For this review, take the finished solid that the model builds, in its own axes (mm). Face numbers are marked on the shaded views. Give positions to 0.01 mm unless a question says otherwise; leave off trailing zeros. Order: outer loops, then holes, each group sorted by start corner. A loop starts at its lowest first (then second) coordinate and runs counter-clockwise, first axis right, second up. Notation, with made-up numbers: (89, -16.75) - (100, -16.75) arc R27 ccw to (100, 17.25) - close; hole circle Ø1 at (47.25, -7.75). An arc over 180 degrees is marked (long way). Use a Markdown table: item, result. Add a question column.
1) Clearance check with flat-ended pins moving along their axes: P1, Ø5, axis at y = 17.5, z = 117.5, coming from the +X side; P2, Ø1, axis at y = 23, z = 14.5, coming from the +X side; P3, Ø4, axis at y = 13.5, z = 117.5, coming from the -X side. State where each tip first meets the part, or that it passes through.
2) We need section C-C on x = 18. Write out the cut boundary in (y, z).
3) We need section D-D on y = 2.5. Write out the cut boundary in (x, z), then the cut area to 3 significant figures.
4) We need section B-B on z = 95. Write out the cut boundary in (x, y), then the cut area to 3 significant figures.
5) Mouldability with a two-part tool opening along Y and no side actions: class the marked faces 1, 2, 3 and 4 as released by +Y, released by -Y, zero draft, split by the parting line, or undercut.
6) We need section A-A on x = 31. Write out the cut boundary in (y, z), then the cut area to 3 significant figures.
7) Wall thickness on L1, parallel to X at y = -12.5, z = 3; L2, parallel to Y at x = 34, z = 69.5; L3, parallel to Y at x = 8, z = 102: over which ranges is each line inside the solid? List them lowest first.
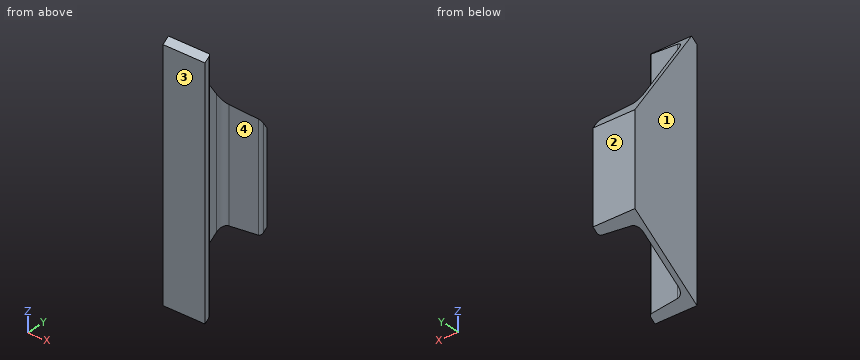
Autodesk Inventor part; units mm, degrees
ref_plane "Начальная плоскость" through (0, 0, -22.1942) normal (0, 0, 1) x (1, 0, 0)
ref_plane "Конечная плоскость" through (0, 0, 186.7165) normal (0, 0, 1) x (1, 0, 0)
ref_plane "РабПлоскость8" through (-29, 0, 205.1172) normal (0, -0.5661745, 0.8242854) x (1, 0, 0)
ref_plane "Начальная плоскость" through (0, 0, -22.1942) normal (0, 0, 1) x (1, 0, 0)
ref_plane "Конечная плоскость" through (0, 0, 186.7165) normal (0, 0, 1) x (1, 0, 0)
sketch "Эскиз" plane through (0, 0, 0) normal (0, 0, 1) x (1, 0, 0)
  line L0 (36, -32.5) -> (0, -32.5)
  line L1 (36, -32.5) -> (36, -28.696)
  line L2 (33.6994, -26.2039) -> (9.9215, -24.3017)
  line L3 (4.4, -18.3208) -> (4.4, 18.3208)
  line L4 (33.6994, 26.2039) -> (9.9215, 24.3017)
  line L5 (36, 28.696) -> (36, 32.5)
  line L6 (0, 32.5) -> (36, 32.5)
  line L7 (0, -32.5) -> (0, 32.5)
  arc A0 (4.4, -18.3208) -> (9.9215, -24.3017) centre (10.4, -18.3208) ccw
  arc A1 (9.9215, 24.3017) -> (4.4, 18.3208) centre (10.4, 18.3208) ccw
  arc A2 (36, -28.696) -> (33.6994, -26.2039) centre (33.5, -28.696) ccw
  arc A3 (33.6994, 26.2039) -> (36, 28.696) centre (33.5, 28.696) ccw
  line L8 (0, 45.5) -> (0, -45.5) construction
  line L9 (-7.2974, 0) -> (43.7847, 0) construction
  point P0 (36, -26.388)
  point P1 (4.4, -23.86)
  point P2 (4.4, 23.86)
  point P3 (36, 26.388)
  dimension "d3" = 36
  dimension "d5" = 4.4
  dimension "d7" = 65
  dimension "d9" = 8.64
  dimension "d11" = 8.64
  dimension "d13" = 6.112
  dimension "d15" = 6.112
  dimension "d22" = 6
  dimension "d23" = 2.5
  dimension "d24" = 32.5
  dimension "d25" = 0
extrude "Тело" add sketch "Эскиз" along normal up to surface (208.9107 mm away) from surface at -22.1942
sketch "Sketch3" plane through (0, 0, 0) normal (0, 0, 1) x (1, 0, 0)
  line L0 (0, 0) -> (10, 0)
ref_plane "Work Plane7" through (0, 0, 0) normal (0, -1, 0) x (1, 0, 0)
sketch "Sketch4" plane through (0, 0, 0) normal (0, -1, 0) x (1, 0, 0)
  line L0 (-2, -22.1942) -> (12, -22.1942)
  line L1 (-2, 186.7165) -> (12, 186.7165)
  dimension "d29" = 208.9107
ref_plane "РабПлоскость8" through (-29, 0, 205.1172) normal (0, -0.5661745, 0.8242854) x (1, 0, 0)
split "Разделение1" plane through (-29, 0, 205.1172) removes the side toward (0, -0.5661745, 0.8242854)
ref_plane "РабПлоскость9" through (36, 328.8626, 224.5798) normal (0, 0.5639457, -0.8258119) x (1, 0, 0)
split "Разделение2" plane through (36, 328.8626, 224.5798) removes the side toward (0, 0.5639457, -0.8258119)
ref_plane "РабПлоскость10" through (36, 68.6864, 46.906) normal (0, 0.8258135, 0.5639433) x (1, 0, 0)
split "Разделение3" plane through (36, 68.6864, 46.906) removes the side toward (0, 0.8258135, 0.5639433)
equation "\"d3\" = b"
equation "\"d7\" = ParH"
equation "\"d22\" = R"
equation "\"d23\" = R1"
equation "\"d24\" = 0.5 * d7"
equation "\"d16\" = G_L"
equation "\"R1\" = 2.5"
equation "\"R\" = 6"
equation "\"t1\" = 4.4"
equation "\"t2\" = 7.2"
equation "\"ParH\" = 65"
equation "\"b\" = 36"
equation "\"msp_x1\" = 0.04 * b"
equation "\"msp_x2\" = -0.08 * t1 + 0.04 * b"
equation "\"G_L\" = d29"
equation "\"ex\" = 0"
equation "\"G_OFFSET_START\" = 22.1942"
equation "\"G_OFFSET_END\" = -18.40074"
equation "\"d26\" = -G_OFFSET_START"
equation "\"d27\" = G_OFFSET_END + B_L"
equation "\"B_L\" = 205.11724"
properties part number "Швеллер 6.5U-208,91 ГОСТ 8240-97" material "Сталь, мягкая"
Checked values:
| question | item | result |
|---|---|---|
| 1 | P1 | x = 4.64 |
| 1 | P2 | through |
| 1 | P3 | x = 0 |
| 2 | outline | (-32.5, -22.19) - (-24.95, -17.04) - (-24.95, 184.02) - (-26.79, 186.72) - (-32.5, 182.79) - close; (24.95, 17.04) - (32.5, 22.19) - (32.5, 99.9) - (24.95, 110.95) - close |
| 3 | outline | (0, 1.71) - (4.4, 1.71) - (4.4, 143.83) - (0, 143.83) - close |
| 3 | area | 625 mm² |
| 4 | outline | (0, -32.5) - (36, -32.5) - (36, -28.7) arc R2.5 ccw to (33.7, -26.2) - (9.92, -24.3) arc R6 cw to (4.4, -18.32) - (4.4, 18.32) arc R6 cw to (9.92, 24.3) - (33.7, 26.2) arc R2.5 ccw to (36, 28.7) - (36, 32.5) - (0, 32.5) - close |
| 4 | area | 763 mm² |
| 5 | face 1 | zero draft |
| 5 | face 2 | released by +Y |
| 5 | face 3 | released by -Y |
| 5 | face 4 | undercut |
| 6 | outline | (-32.5, -22.19) - (-25.99, -17.75) - (-25.99, 185.54) - (-26.79, 186.72) - (-32.5, 182.79) - close; (25.99, 17.75) - (32.5, 22.19) - (32.5, 99.9) - (25.99, 109.43) - close |
| 6 | area | 1,890 mm² |
| 7 | L1 | 0 to 4.4 |
| 7 | L2 | -32.5 to -26.25, 26.25 to 32.5 |
| 7 | L3 | -32.5 to -23.82, 23.82 to 31.06 |
